Verification items for the finished model (mm, model axes). A direction names the side the tool comes from. Give positions to 0.01 mm unless a question says otherwise; leave off trailing zeros. Order: outer loops, then holes, each group sorted by start corner. A loop starts at its lowest first (then second) coordinate and runs counter-clockwise, first axis right, second up.
from build123d import *
from build123d.topology import SkipClean

# Parameters (mm, degrees)
BOSS_EXTRUDE1_DEPTH   = 10
SKETCH2_R             = 26
BOSS_EXTRUDE2_DEPTH   = 15
SKETCH3_R             = 55
SKETCH3_R_2           = 44
BOSS_EXTRUDE3_DEPTH   = 15
EXTRUDE_THIN1_START   = -15
EXTRUDE_THIN1_DEPTH   = 15
EXTRUDE_THIN2_START   = -15
EXTRUDE_THIN2_DEPTH   = 15
F_1_0MM_DOWEL_HOLE1_D = 40


# Read off the part's stored shape, not the designer's step: Extrude-Thin1, Extrude-Thin2
with BuildPart() as part:
    # Sketch1 → Boss-Extrude1 (new body)
    with BuildSketch(Plane(origin=(0, 0, 0), x_dir=(1, 0, 0), z_dir=(0, 1, 0))):
        with BuildLine():
            Line((18.384776311, -131.384776311), (131.384776311, -18.384776311))
            ThreePointArc((131.384776311, -18.384776311), (134.295069945, 14.917104144), (102.002815768, 23.559752524))
            ThreePointArc((102.002815768, 23.559752524), (74.773631801, 21.15717706), (52.359428182, 36.803400392))
            ThreePointArc((52.359428182, 36.803400392), (45.254833996, 45.254833996), (36.803400392, 52.359428182))
            ThreePointArc((36.803400392, 52.359428182), (21.15717706, 74.773631801), (23.559752524, 102.002815768))
            ThreePointArc((23.559752524, 102.002815768), (0, 139), (-23.559752524, 102.002815768))
            ThreePointArc((-23.559752524, 102.002815768), (-21.15717706, 74.773631801), (-36.803400392, 52.359428182))
            ThreePointArc((-36.803400392, 52.359428182), (-45.254833996, 45.254833996), (-52.359428182, 36.803400392))
            ThreePointArc((-52.359428182, 36.803400392), (-74.773631801, 21.15717706), (-102.002815768, 23.559752524))
            ThreePointArc((-102.002815768, 23.559752524), (-134.295069945, 14.917104144), (-131.384776311, -18.384776311))
            Line((-131.384776311, -18.384776311), (-18.384776311, -131.384776311))
            ThreePointArc((-18.384776311, -131.384776311), (0, -139), (18.384776311, -131.384776311))
        make_face()
    extrude(amount=BOSS_EXTRUDE1_DEPTH)

    # Sketch2 → Boss-Extrude2 (add)
    with BuildSketch(Plane(origin=(0, 10, 0), x_dir=(1, 0, 0), z_dir=(0, 1, 0))):
        with Locations(Location((0, 113, 0), (0, 0, 205.022151532))):
            Circle(SKETCH2_R)
        with Locations(Location((113, 0, 0), (0, 0, 115.022151532))):
            Circle(SKETCH2_R)
        with Locations(Location((-113, 0, 0), (0, 0, 64.977848468))):
            Circle(SKETCH2_R)
        with Locations(Location((0, -113, 0), (0, 0, 315))):
            Circle(SKETCH2_R)
    extrude(amount=BOSS_EXTRUDE2_DEPTH)

    # Sketch3 → Boss-Extrude3 (add)
    with BuildSketch(Plane(origin=(0, 10, 0), x_dir=(1, 0, 0), z_dir=(0, 1, 0))):
        with Locations(Location((0, 0, 0), (0, 0, 270))):
            Circle(SKETCH3_R)
        with Locations(Location((0, 0, 0), (0, 0, 270))):
            Circle(SKETCH3_R_2, mode=Mode.SUBTRACT)
    extrude(amount=BOSS_EXTRUDE3_DEPTH)

    # Extrude-Thin1 outline → Extrude-Thin1 (add)
    with SkipClean():  # the faces are left unmerged after this step: merging them gives an invalid solid
        with BuildSketch(Plane(origin=(0, 25, 0), x_dir=(1, 0, 0), z_dir=(0, 1, 0)).offset(EXTRUDE_THIN1_START)):
            with BuildLine():
                Line((-89, -10), (-54.083269132, -10))
                ThreePointArc((-54.083269132, -10), (-54.770337785, -5.02096593), (-55, 0))
                Line((-55, 0), (-87, 0))
                ThreePointArc((-87, 0), (-87.504902432, -5.099019514), (-89, -10))
            make_face()
            with BuildLine():
                ThreePointArc((10, -54.083269132), (0, -55), (-10, -54.083269132))
                Line((-10, -54.083269132), (-10, -89))
                ThreePointArc((-10, -89), (0, -87), (10, -89))
                Line((10, -89), (10, -54.083269132))
            make_face()
            with BuildLine():
                Line((87, 0), (55, 0))
                ThreePointArc((55, 0), (54.770337785, -5.02096593), (54.083269132, -10))
                Line((54.083269132, -10), (89, -10))
                ThreePointArc((89, -10), (87.504902432, -5.099019514), (87, 0))
            make_face()
        extrude(amount=EXTRUDE_THIN1_DEPTH)

    # Extrude-Thin2 outline → Extrude-Thin2 (add)
    with SkipClean():  # the faces are left unmerged after this step: merging them gives an invalid solid
        with BuildSketch(Plane(origin=(0, 25, 0), x_dir=(1, 0, 0), z_dir=(0, 1, 0)).offset(EXTRUDE_THIN2_START)):
            with BuildLine():
                Line((89, 10), (54.083269132, 10))
                ThreePointArc((54.083269132, 10), (54.770337785, 5.02096593), (55, 0))
                Line((55, 0), (87, 0))
                ThreePointArc((87, 0), (87.504902432, 5.099019514), (89, 10))
            make_face()
            with BuildLine():
                ThreePointArc((-55, 0), (-54.770337785, 5.02096593), (-54.083269132, 10))
                Line((-54.083269132, 10), (-89, 10))
                ThreePointArc((-89, 10), (-87.504902432, 5.099019514), (-87, 0))
                Line((-87, 0), (-55, 0))
            make_face()
            with BuildLine():
                Line((-10, 89), (-10, 54.083269132))
                ThreePointArc((-10, 54.083269132), (0, 55), (10, 54.083269132))
                Line((10, 54.083269132), (10, 89))
                ThreePointArc((10, 89), (0, 87), (-10, 89))
            make_face()
        extrude(amount=EXTRUDE_THIN2_DEPTH)

    # Ø1.0mm Dowel Hole1 (through all)
    with Locations(Plane(origin=(0, 25, 0), x_dir=(1, 0, 0), z_dir=(0, 1, 0))):
        with Locations((0, 113), (-113, 0), (113, 0), (0, -113)):
            Hole(F_1_0MM_DOWEL_HOLE1_D / 2)


solid = part.part
(1) Release check for a two-part mould opening along Z. For faces 4 (the cylindrical face through (4.336, 12.325, 132.524)), 5 (the flat face through (-32, 25, -32)), 6 (the flat face through (72, 17, -10)), 7 (the cylindrical face through (21.26, 4.93, -74.4)) record: pulls with the +Z half, pulls with the -Z half, needs draft (parallel to the pull), parting line crosses it, or undercut.
Solved:
face 4: undercut
face 5: needs draft
face 6: pulls with the -Z half
face 7: undercut
(2) Scan lines: line 1 (X direction, y = 19.25, z = -1.5); line 2 (Z direction, x = -113, y = 18.25). Record each from-to range of solid material in increasing order.
Solved:
line 1: x = -138.96 to -132.94, -93.06 to -43.97, 43.97 to 93.06, 132.94 to 138.96
line 2: z = -26 to -20, 20 to 26
(3) Go/stop test with flat-tipped pins: pin 1 (4 mm diameter, centred on x = -52, y = 19, fed in from -Z); pin 2 (7.5 mm diameter, centred on y = 19.5, z = 76.5, fed in from -X); pin 3 (7.5 mm diameter, centred on y = 14.5, z = 65, fed in from +X). Record where each tip stops, or that it passes through.
Solved:
pin 1: stops at z = -22.91
pin 2: stops at x = -10
pin 3: stops at x = 10
(4) Set-up check for faces 1 (the flat face through (42, 10, -46)), 2 (the flat face through (71, 17, 10)), 3 (the flat face through (10, 17, -71)): record each of +Z, -Z, +X, -X, +Y, -Y from which the full face is reachable in a straight line by a thin tool's end or side.
Solved:
face 1: +Y
face 2: +Z, +Y
face 3: +X, +Y
(5) Section check C-C, the plane x = 114. Enter the section's corners in (y, z), then the cut area to 3 significant figures.
Solved:
outline: (0, -25.98) - (25, -25.98) - (25, -19.97) - (0, -19.97) - close; (0, 19.97) - (25, 19.97) - (25, 25.98) - (10, 25.98) - (10, 35.77) - (0, 35.77) - close
area: 398 mm2
(6) Section check B-B, the plane z = -113. Enter the section's corners in (x, y), then the cut area to 3 significant figures.
Solved:
outline: (-26, 0) - (-20, 0) - (-20, 25) - (-26, 25) - close; (20, 0) - (26, 0) - (26, 25) - (20, 25) - close
area: 300 mm2
(7) Section check A-A, the plane z = 0. Enter the section's corners in (x, y), then the cut area to 3 significant figures.
Solved:
outline: (-139, 0) - (-133, 0) - (-133, 25) - (-139, 25) - close; (-93, 0) - (93, 0) - (93, 25) - (44, 25) - (44, 10) - (-44, 10) - (-44, 25) - (-93, 25) - close; (133, 0) - (139, 0) - (139, 25) - (133, 25) - close
area: 3,630 mm2
(8) Section check D-D, the plane y = 19. Enter the section's corners in (x, z), then the cut area to 3 significant figures.
Solved:
outline: (-89, -10) - (-54.08, -10) arc R55 ccw to (-10, -54.08) - (-10, -89) arc R26 ccw (long way) to (10, -89) - (10, -54.08) arc R55 ccw to (54.08, -10) - (89, -10) arc R26 ccw (long way) to (89, 10) - (54.08, 10) arc R55 ccw to (10, 54.08) - (10, 89) arc R26 ccw (long way) to (-10, 89) - (-10, 54.08) arc R55 ccw to (-54.08, 10) - (-89, 10) arc R26 ccw (long way) to start; hole circle Ø40 at (-113, 0); hole circle Ø88 at (0, 0); hole circle Ø40 at (0, -113); hole circle Ø40 at (0, 113); hole circle Ø40 at (113, 0)
area: 9,530 mm2
